Can you work these out from the model? Positions are in its coordinate system, mm. A direction names the side the tool comes from. Coordinates: 2 decimals unless noted, no trailing zeros. Order: outer loops, then holes, each group sorted by start corner. A loop starts at its lowest first (then second) coordinate and runs counter-clockwise, first axis right, second up. Notation, with made-up numbers: (9.25, 29) - (54.25, 29) arc R17 ccw to (54.25, 36) - close; hole circle Ø10 at (-7.5, 4). An arc over 180 degrees is marked (long way). Return JSON: item names as keys, results as strings. Group by question number.
1) Imagine slicing it at B-B (x = 0). Write out the boundary of the cut face in (y, z).
2) Imagine slicing it at D-D (z = 9.5). Write out the boundary of the cut face in (x, y), and give its area (3 significant figures).
3) Imagine slicing it at C-C (y = 2). Write out the boundary of the cut face in (x, z).
4) If I drill on line 1 along Z through (x, y) = (1, 3); line 2 along X through (y, z) = (0.5, 1); line 3 along Y through (x, z) = (-0.5, 7), over which ranges is the centre line in solid material (lowest first)?
5) For pin 1 Ø1.5 at (x, z) = (-0.5, 4.5) entering from -Y; pin 2 Ø1 at (x, z) = (0.5, 9) entering from -Y, each with a flat end and sliding along its axis, tell me the tip position at first contact or that it passes through.
6) Imagine slicing it at A-A (z = 2). Write out the boundary of the cut face in (x, y), and give its area (3 significant figures).
7) Which directions (+Z, -Z, +X, -X, +Y, -Y) give clear straight access to the entire face, cutting with the end or side of a thin tool? Please do faces 1 (the face through (-2, 2, 4)), 2 (the face through (4.29, -1.44, 1.97)).
```python
from build123d import *

# Parameters (mm, degrees)
SKETCH1_R           = 2.5
BOSS_EXTRUDE3_DEPTH = 4
SKETCH2_R           = 2.5
BOSS_EXTRUDE4_DEPTH = 13


with BuildPart() as part:
    # Sketch1 → Boss-Extrude3 (new body)
    with BuildSketch(Plane.XY):
        Polygon((3.493859283, -3.885138771), (5.111558514, 1.08320151), (1.617699232, 4.968340281), (-3.493859283, 3.885138771), (-5.111558514, -1.08320151), (-1.617699232, -4.968340281), align=None)
        Circle(SKETCH1_R, mode=Mode.SUBTRACT)
    extrude(amount=BOSS_EXTRUDE3_DEPTH)

    # Sketch2 → Boss-Extrude4 (add)
    with BuildSketch(Plane(origin=(0, 0, 0), x_dir=(-1, 0, 0), z_dir=(0, 0, -1))):
        Circle(SKETCH2_R)
    extrude(amount=-BOSS_EXTRUDE4_DEPTH)


solid = part.part
```
Calculated:
{
 "1": {"outline": "(-4.63, 0) - (4.63, 0) - (4.63, 4) - (2.5, 4) - (2.5, 13) - (-2.5, 13) - (-2.5, 4) - (-4.63, 4) - close"},
 "2": {"outline": "circle Ø5 at (0, 0)", "area": "19.6 mm2"},
 "3": {"outline": "(-4.11, 0) - (4.29, 0) - (4.29, 4) - (1.5, 4) - (1.5, 13) - (-1.5, 13) - (-1.5, 4) - (-4.11, 4) - close"},
 "4": {"line 1": "0 to 4", "line 2": "-4.6 to 4.92", "line 3": "-2.45 to 2.45"},
 "5": {"pin 1": "y = -4.85", "pin 2": "y = -2.5"},
 "6": {"outline": "(-5.11, -1.08) - (-1.62, -4.97) - (3.49, -3.89) - (5.11, 1.08) - (1.62, 4.97) - (-3.49, 3.89) - close", "area": "70.9 mm2"},
 "7": {"face 1": "+Z", "face 2": "+Z, -Z, +X, -Y"}
}
